Could you check a few things on this drawing? It's one solid part, dimensions in mm from its lowest x, y, z. A direction names the side the tool comes from. Give positions to 0.01 mm unless a question says otherwise; leave off trailing zeros. Write each loop counter-clockwise with the first axis right and the second up, starting at its lowest first coordinate (ties: lowest second). Pieces come first, ordered by that corner, then holes. Notation, with made-up numbers: M -17,86.5 L 7,86.5 A21 ccw 7,91.5 Z; hole C 63,63 d2. An arc over 180 degrees is marked long. Answer as CSV lines item,"result". Start each with the question number.
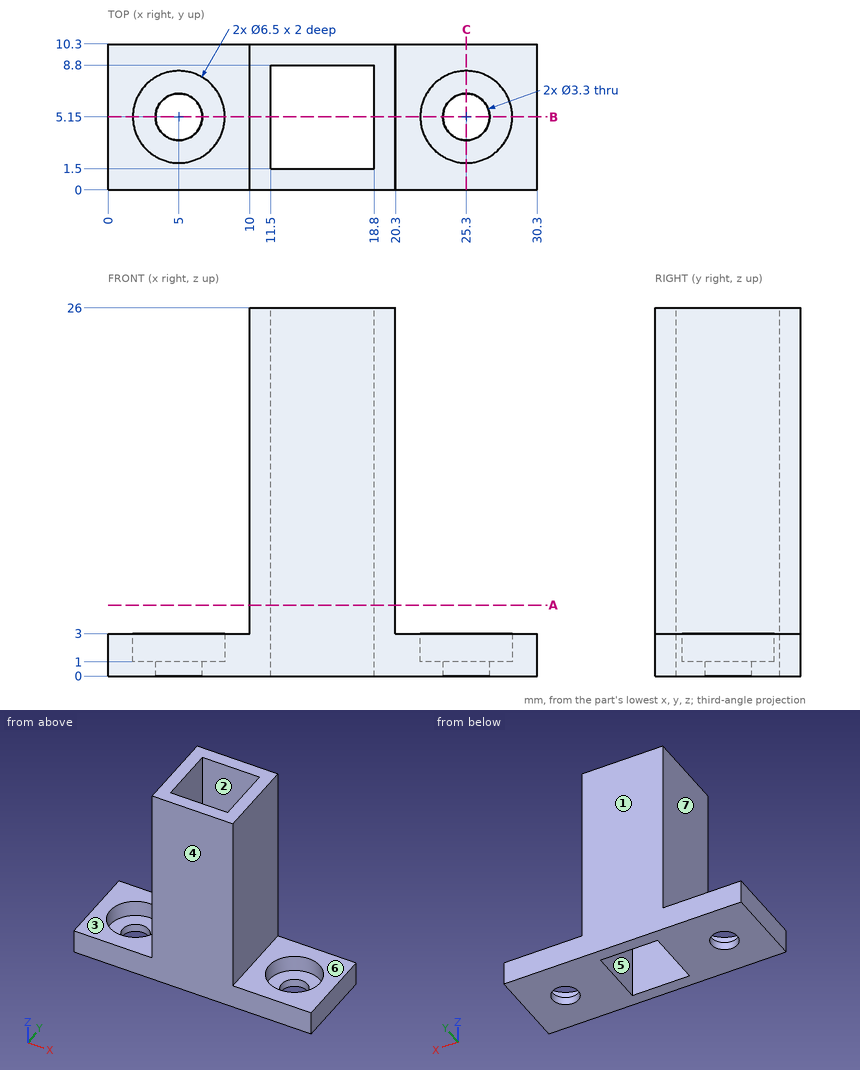
1) I want a section at B-B, the plane y = 5.15. Please give me the cut outline in (x, z), then the cut area to 3 significant figures.
2) Thinking about a two-plate mould opening in Y: for the marked faces 1, 2, 3 and 4, which applies, released by +Y, released by -Y, zero draft, split by the parting line, or undercut?
3) I want a section at C-C, the plane x = 25.3. Please give me the cut outline in (y, z), then the cut area to 3 significant figures.
4) On a 3-axis mill with a long thin cutter (end or side, diameter ignored), from which of +Z, -Z, +X, -X, +Y, -Y can I reach the whole of each face in a straight line? I mean the marked faces 5, 6 and 7. Say none if no direction works.
5) I want a section at A-A, the plane z = 5. Please give me the cut outline in (x, y), then the cut area to 3 significant figures.
6) I'm going to push flat-ended pins straight in: P1, Ø1.5, axis at y = 3.5, z = 15.5, coming from the -X side; P2, Ø4, axis at x = 23.5, y = 3, coming from the +Z side; P3, Ø3, axis at x = 25.5, y = 6, coming from the +Z side. Where does each tip first touch, or does it pass through?
7) I need wall thicknesses on L1, parallel to X at y = 5.15, z = 0.3; L2, parallel to X at y = 8, z = 13; L3, parallel to Z at x = 3, y = 4. Which ranges of each line are inside material? Lowest first, please. Write a range as from..to.
Values found:
1,outline,"M 0,0 L 3.35,0 L 3.35,1 L 1.75,1 L 1.75,3 L 0,3 Z; M 6.65,0 L 11.5,0 L 11.5,26 L 10,26 L 10,3 L 8.25,3 L 8.25,1 L 6.65,1 Z; M 18.8,0 L 23.65,0 L 23.65,1 L 22.05,1 L 22.05,3 L 20.3,3 L 20.3,26 L 18.8,26 Z; M 26.95,0 L 30.3,0 L 30.3,3 L 28.55,3 L 28.55,1 L 26.95,1 Z"
1,area,"105 mm²"
2,face 1,"released by +Y"
2,face 2,"undercut"
2,face 3,"zero draft"
2,face 4,"released by -Y"
3,outline,"M 0,0 L 3.5,0 L 3.5,1 L 1.9,1 L 1.9,3 L 0,3 Z; M 6.8,0 L 10.3,0 L 10.3,3 L 8.4,3 L 8.4,1 L 6.8,1 Z"
3,area,"14.6 mm²"
4,face 5,"+Z, -Z"
4,face 6,"+Z, +X, +Y, -Y"
4,face 7,"+Z, -X, +Y, -Y"
5,outline,"M 10,0 L 20.3,0 L 20.3,10.3 L 10,10.3 Z; hole M 11.5,1.5 L 18.8,1.5 L 18.8,8.8 L 11.5,8.8 Z"
5,area,"52.8 mm²"
6,P1,"stops at x = 10"
6,P2,"stops at z = 3"
6,P3,"stops at z = 1"
7,L1,"x = 0..3.35, 6.65..11.5, 18.8..23.65, 26.95..30.3"
7,L2,"x = 10..11.5, 18.8..20.3"
7,L3,"z = 0..1"
